Could you check a few things on this model? Use its own coordinates, in mm. Round coordinates to 2 decimals unless told otherwise and drop trailing zeros. Loops run counter-clockwise (first coordinate to the right, second up) from the corner with the lowest first, then second, coordinate; pieces in that order, holes last. Notation, with made-up numbers: (55, 68) -> (79, 68) arc R28 cw to (79, 102) -> close; hole circle Ø11 at (-20.75, 4). An arc over 180 degrees is marked (long way). One line per item, written item: value.
```python
from build123d import *

# Parameters (mm, degrees)
SKETCH1_W           = 498.348
SKETCH1_H           = 165.1
BOSS_EXTRUDE1_DEPTH = 1.143
SKETCH2_W           = 69.85
SKETCH2_H           = 2.286
BOSS_EXTRUDE2_DEPTH = 3.175
LPATTERN1_COUNT     = 5
LPATTERN1_PITCH     = 98.8568


with BuildPart() as part:
    # Sketch1 → Boss-Extrude1 (new, symmetric)
    with BuildSketch(Plane(origin=(0, 0, 0), x_dir=(1, 0, 0), z_dir=(0, 1, 0))):
        Rectangle(SKETCH1_W, SKETCH1_H)
    extrude(amount=BOSS_EXTRUDE1_DEPTH, both=True)

    # Sketch2 → Boss-Extrude2 (add)
    with BuildSketch(Plane(origin=(0, 0, -82.55), x_dir=(-1, 0, 0), z_dir=(0, 0, -1))):
        with Locations((-197.7136, 0)):
            Rectangle(SKETCH2_W, SKETCH2_H)
    boss_extrude2 = extrude(amount=BOSS_EXTRUDE2_DEPTH)

    # LPattern1: Boss-Extrude2 ×5
    with Locations(*[(-i * LPATTERN1_PITCH, 0, 0) for i in range(1, LPATTERN1_COUNT)]):
        add(boss_extrude2)


solid = part.part
```
Item 1: Will these pins go through, and if not, where does the flat tip stop? pin 1 Ø1.1 at (y, z) = (0.5, -84.5) entering from +X; pin 2 Ø0.7 at (x, y) = (-245, 0) entering from -Z; pin 3 Ø0.7 at (y, z) = (-0.5, -84.5) entering from -X.
Output:
pin 1: stops at x = 232.64
pin 2: stops at z = -82.55
pin 3: stops at x = -232.64
Item 2: If we section it at A-A on x = -46.5: List the corners of the cut face in (y, z) for me, plus the area to 3 significant figures.
Output:
outline: (-1.14, -82.55) -> (1.14, -82.55) -> (1.14, 82.55) -> (-1.14, 82.55) -> close
area: 377 mm²
Item 3: I need wall thicknesses on line 1 (Z direction, x = -137, y = -0.85). Which ranges of the line are inside material? Lowest first, please. Write a range as from..to.
Output:
line 1: z = -82.55..82.55
